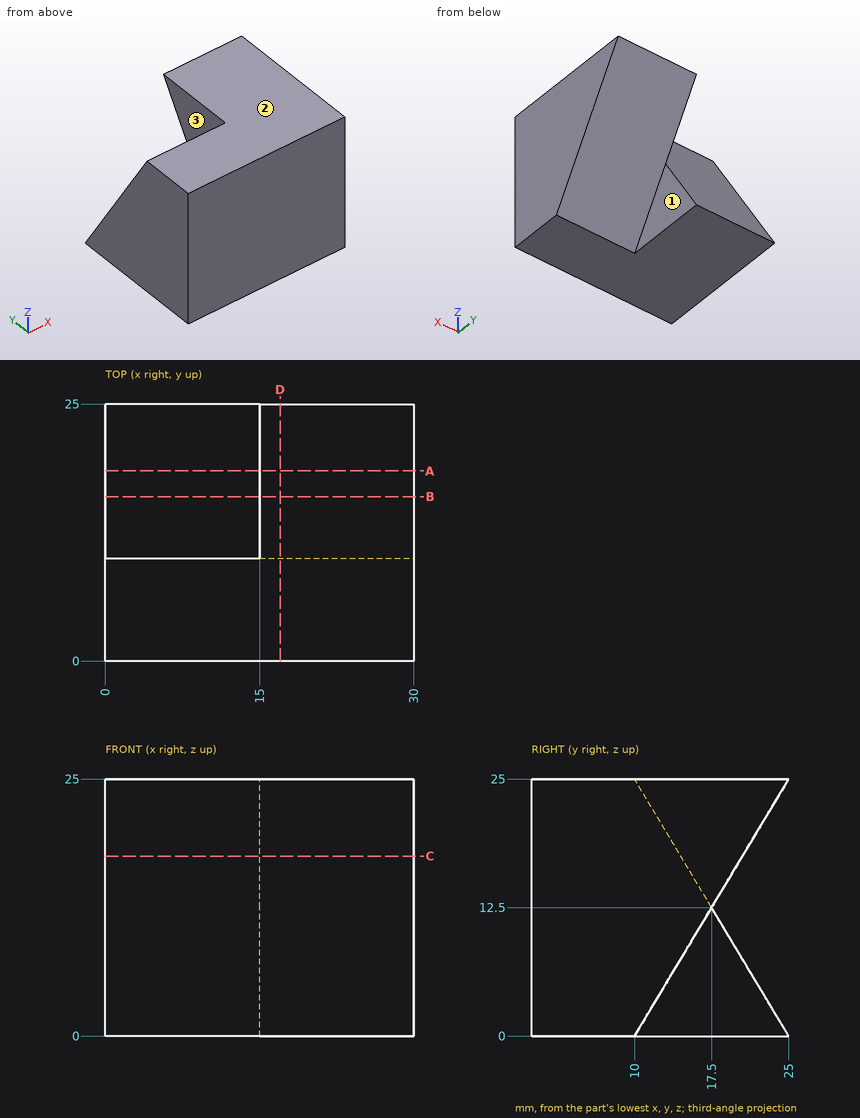
Can you work these out from the drawing? Everything is in mm from the part's minimum corner. A direction names the side the tool comes from. Coordinates: 2 decimals unless noted, no trailing zeros. Order: outer loops, then holes, each group sorted by start corner. A loop starts at its lowest first (then second) coordinate and runs counter-clockwise, first axis right, second up. Notation, with made-up numbers: (4.5, -33) -> (53.5, -33) arc R16 cw to (53.5, -9) -> close; hole circle Ø11 at (7, -23). An arc over 180 degrees is marked (long way). Use one line per item in the form item = value.
Q1. Imagine slicing it at D-D, the plane x = 17. List the corners of the cut face in (y, z) for me, then the cut area to 4 significant figures.
From the geometry:
outline = (0, 0) -> (10, 0) -> (25, 25) -> (0, 25) -> close
area = 437.5 mm²
Q2. Which directions (+Z, -Z, +X, -X, +Y, -Y) give clear straight access to the entire face, cutting with the end or side of a thin tool? Please do the marked faces 1, 2 and 3.
From the geometry:
face_1 = -Z, +X, +Y
face_2 = +Z, +X, -X, +Y, -Y
face_3 = +Z, -X, +Y
Q3. I need wall thicknesses on L1, parallel to X at y = 14.5, z = 3.75; L2, parallel to Z at x = 25.25, y = 19; L3, parallel to Z at x = 25.75, y = 15. Which ranges of each line are inside material? Lowest first, please.
From the geometry:
L1 = 0 to 15
L2 = 15 to 25
L3 = 8.33 to 25
Q4. Imagine slicing it at C-C, the plane z = 17.5. List the corners of the cut face in (x, y) for me, then the cut area to 3 significant figures.
From the geometry:
outline = (0, 0) -> (30, 0) -> (30, 20.5) -> (15, 20.5) -> (15, 14.5) -> (0, 14.5) -> close
area = 525 mm²
Q5. Will these pins go through, and if not, where does the flat tip stop? P1, Ø6, axis at x = 16, y = 8.5, coming from the -Z side; P2, Ø5, axis at x = 12, z = 14.5, coming from the +Y side; P3, Ø1, axis at x = 17, y = 21, coming from the -Z side; P4, Ø4, axis at y = 17.5, z = 20, coming from the -X side.
From the geometry:
P1 = 0
P2 = 17.8
P3 = 17.5
P4 = 15
Q6. Imagine slicing it at A-A, the plane y = 18.5. List the corners of the cut face in (x, z) for me, then the cut area to 3 significant figures.
From the geometry:
outline = (0, 0) -> (15, 0) -> (15, 10.83) -> (0, 10.83) -> close; (15, 14.17) -> (30, 14.17) -> (30, 25) -> (15, 25) -> close
area = 325 mm²
Q7. Imagine slicing it at B-B, the plane y = 16. List the corners of the cut face in (x, z) for me, then the cut area to 3 significant figures.
From the geometry:
outline = (0, 0) -> (15, 0) -> (15, 10) -> (30, 10) -> (30, 25) -> (15, 25) -> (15, 15) -> (0, 15) -> close
area = 450 mm²
